Here's how the part is built. I have some questions about the finished solid (model axes, mm). A direction names the side the tool comes from. Give positions to 0.01 mm unless a question says otherwise; leave off trailing zeros. Write each loop counter-clockwise with the first axis right and the second up, starting at its lowest first coordinate (ties: lowest second). Pieces come first, ordered by that corner, then holes. Notation, with made-up numbers: (-7.75, -26.5) -> (49.25, -26.5) arc R15 ccw to (49.25, -7.5) -> close; hole circle Ø3 at (43, 32.5). An arc over 180 degrees is marked (long way). Put each result on its own line as item: value. Start each with the question number.
from build123d import *

# Parameters (mm, degrees)
F0_W      = 110
F0_H      = 110
F1_DEPTH  = 5
F3_DEPTH  = 100
F4_SIZE   = 7
F6_DEPTH  = 5
F8_DEPTH  = 100
F9_R      = 3
F10_R     = 3
F11_R     = 5
F12_R     = 40
F13_DEPTH = 2
F14_R     = 40
F15_DEPTH = 2


with BuildPart() as f1:
    # F0 (on Top) → F1 (new body)
    with BuildSketch(Plane.XY):
        Rectangle(F0_W, F0_H)
    extrude(amount=F1_DEPTH)

    # F2 (on face) → F3 (join)
    with BuildSketch(Plane.XY.offset(5)):
        Polygon((-55, -45), (-55, -55), (-45, -55), (-45, -50), (-50, -50), (-50, -45), align=None)
        Polygon((45, -50), (45, -55), (55, -55), (55, -45), (50, -45), (50, -50), align=None)
        Polygon((50, 45), (55, 45), (55, 55), (45, 55), (45, 50), (50, 50), align=None)
        Polygon((-55, 45), (-50, 45), (-50, 50), (-45, 50), (-45, 55), (-55, 55), align=None)
    extrude(amount=F3_DEPTH)

    # F4
    f4_edges = [f1.edges().sort_by_distance(p)[0] for p in [
        (55, -55, 52.5),
        (55, 55, 52.5),
        (-55, -55, 52.5),
        (-55, 55, 52.5),
    ]]
    chamfer(f4_edges, length=F4_SIZE)

    # F5 (on face) → F6 (join)
    with BuildSketch(Plane(origin=(0, 0, 0), x_dir=(1, 0, 0), z_dir=(0, 0, -1))):
        Polygon((-55, -48), (-55, 48), (-86.8553390593, 16.1446609407), (-86.8553390593, -86.8553390593), (16.1446609407, -86.8553390593), (48, -55), (-48, -55), align=None)
    extrude(amount=-F6_DEPTH)

    # F7 (on face) → F8 (join)
    with BuildSketch(Plane.XY.offset(5)):
        with BuildLine():
            Line((-86.8553390593, -16.1446609407), (-55, -48))
            Line((-55, -48), (-55, -45))
            add(Edge.make_bspline(
                [(-55, -45), (-61.680716385, -38.545717713), (-73.8128115293, -26.9133031572), (-84.5587400556, -12.5278182858), (-85.5100929907, -5.3594725865), (-85.6892368288, -2.2746161558)],
                knots=[0, 0, 0, 0, 0.4166944434, 0.7503780711, 1, 1, 1, 1], degree=3))
            Line((-85.6892368288, -2.2746161558), (-85.6892368288, 84.628576657))
            Line((-85.6892368288, 84.628576657), (-52.0303300859, 50.9696699141))
            Line((-52.0303300859, 50.9696699141), (-50.9696699141, 52.0303300859))
            Line((-50.9696699141, 52.0303300859), (-84.628576657, 85.6892368288))
            Line((-84.628576657, 85.6892368288), (2.2746161558, 85.6892368288))
            add(Edge.make_bspline(
                [(45, 55), (38.545717713, 61.680716385), (26.9133031572, 73.8128115293), (12.5278182858, 84.5587400556), (5.3594725865, 85.5100929907), (2.2746161558, 85.6892368288)],
                knots=[0, 0, 0, 0, 0.4166944434, 0.7503780711, 1, 1, 1, 1], degree=3))
            Line((45, 55), (48, 55))
            Line((48, 55), (16.1446609407, 86.8553390593))
            Line((16.1446609407, 86.8553390593), (-86.8553390593, 86.8553390593))
            Line((-86.8553390593, 86.8553390593), (-86.8553390593, -16.1446609407))
        make_face()
    extrude(amount=F8_DEPTH)

    # F9
    f9_edges = [f1.edges().sort_by_distance(p)[0] for p in [
        (-50.96967, 52.03033, 55),
        (-52.03033, 50.96967, 55),
    ]]
    fillet(f9_edges, radius=F9_R)

    # F10
    f10_edges = [f1.edges().sort_by_distance(p)[0] for p in [
        (45, 55, 55),
        (-55, -45, 55),
        (-85.689237, 84.628577, 55),
        (-84.628577, 85.689237, 55),
    ]]
    fillet(f10_edges, radius=F10_R)

    # F11
    f11_edges = [f1.edges().sort_by_distance(p)[0] for p in [
        (-86.855339, -16.144661, 52.5),
        (16.144661, 86.855339, 52.5),
    ]]
    fillet(f11_edges, radius=F11_R)

    # F12 (on face) → F13 (cut)
    with BuildSketch(Plane(origin=(0, 86.8553390593, 0), x_dir=(-1, 0, 0), z_dir=(0, 1, 0))):
        with Locations((36.3908729653, 52.5)):
            Circle(F12_R)
    extrude(amount=-F13_DEPTH, mode=Mode.SUBTRACT)

    # F14 (on face) → F15 (cut)
    with BuildSketch(Plane(origin=(-86.8553390593, 0, 0), x_dir=(0, -1, 0), z_dir=(-1, 0, 0))):
        with Locations((-36.3908729653, 52.5)):
            Circle(F14_R)
    extrude(amount=-F15_DEPTH, mode=Mode.SUBTRACT)


solid = f1.part
1) I'm going to push flat-ended pins straight in: pin 1 Ø4 at (x, z) = (46.5, 69) entering from +Y; pin 2 Ø4 at (y, z) = (53, 33) entering from +X; pin 3 Ø5.5 at (y, z) = (47.5, 77.5) entering from -X. Where does each tip first touch, or does it pass through?
2) Which directions (+Z, -Z, +X, -X, +Y, -Y) give clear straight access to the entire face, cutting with the end or side of a thin tool? Please do faces 4 (the flat face through (-45, 52, 54)), 5 (the cylindrical face through (3.57, 86.23, 54.26)), 6 (the flat face through (-16, 14, 5)), 7 (the cylindrical face through (-86.464, -16.012, 51.765)).
3) I need wall thicknesses on probe 1 along X at (y, z) = (54, 100.5); probe 2 along Z at (x, y) = (47, -24.5); probe 3 along X at (y, z) = (2.5, 79.5). Which ranges of each line are inside material? Lowest first, please.
4) I want a section at A-A, the plane y = 3. Write out the boundary of the cut face in (x, z), and give its area (3 significant figures).
5) I want a section at B-B, the plane z = 52.5. State how many separate pieces and enclosed holes the cut face has, and give its area (3 significant figures).
6) Thinking about a two-plate mould opening in Z: for faces 1 (the cylindrical face through (-50.937, 53.273, 55.7)), 2 (the flat face through (-53, 48, 105)), 3 (the cylindrical face through (-86.23, 45.06, 13.45)), which applies, released by +Z, released by -Z, zero draft, split by the parting line, or undercut?
Established:
1. pin 1: stops at y = 58.5
1. pin 2: stops at x = 52
1. pin 3: stops at x = -55
2. face 4: +Z, -Y
2. face 5: +Y
2. face 6: +Z
2. face 7: +Z, -Z, -X, -Y
3. probe 1: x = -86.86 to -85.69, -55.06 to -52.93, -49.01 to -45, 44.99 to 49
3. probe 2: z = 0 to 5
3. probe 3: x = -86.86 to -85.69
4. outline: (-86.86, 0) -> (55, 0) -> (55, 5) -> (-85.69, 5) -> (-85.69, 30.48) -> (-86.86, 30.48) -> close; (-86.86, 74.52) -> (-85.69, 74.52) -> (-85.69, 105) -> (-86.86, 105) -> close
4. area: 775 mm2
5. separate pieces: 4
5. enclosed holes: 0
5. area: 591 mm2
6. face 1: zero draft
6. face 2: released by +Z
6. face 3: undercut
